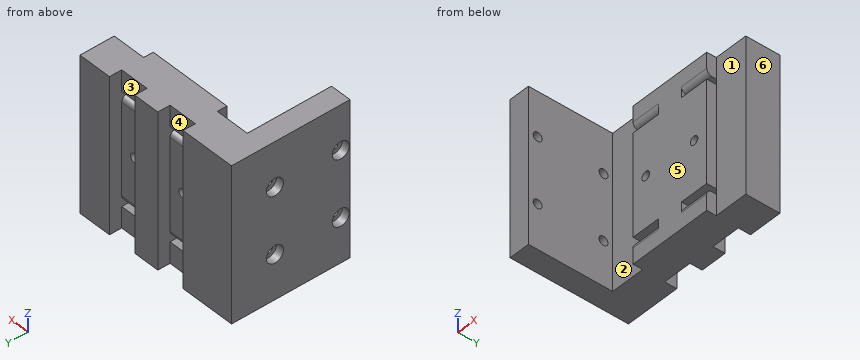
```python
from build123d import *

# Parameters (mm, degrees)
SKETCH1_W                       = 57.8
SKETCH1_H                       = 58.8
BOSS_EXTRUDE1_DEPTH             = 7
SKETCH5_W                       = 57.8
SKETCH5_H                       = 58.8
BOSS_EXTRUDE2_DEPTH             = 6
SKETCH6_W                       = 58.8
SKETCH6_H                       = 45
BOSS_EXTRUDE3_DEPTH             = 8
CBORE_FOR_M3_SHCS2_D            = 3.4
CBORE_FOR_M3_SHCS2_CBORE_D      = 6.5
CBORE_FOR_M3_SHCS2_CBORE_DEPTH  = 3
SKETCH10_W                      = 32
SKETCH10_H                      = 58.8
BOSS_EXTRUDE4_DEPTH             = 3.63
CUT_EXTRUDE1_START              = -4.63
SKETCH11_W                      = 32
SKETCH11_H                      = 8
CUT_EXTRUDE1_DEPTH              = 4.63
SKETCH12_W                      = 32
SKETCH12_H                      = 2
CUT_EXTRUDE2_DEPTH              = 63.094338711
SKETCH17_W                      = 32
SKETCH17_H                      = 58.8
CUT_EXTRUDE3_DEPTH              = 20
BOSS_EXTRUDE5_REACH             = 64.094
SKETCH18_W                      = 10
SKETCH18_H                      = 58.8
BOSS_EXTRUDE5_DIRECTION_2_REACH = 64.094
FILLET1_R                       = 2
M4X0_7_TAPPED_HOLE1_D           = 3.3


with BuildPart() as part:
    # Sketch1 → Boss-Extrude1 (new body)
    with BuildSketch(Plane(origin=(0, 0, 0), x_dir=(1, 0, 0), z_dir=(0, 1, 0))):
        Rectangle(SKETCH1_W, SKETCH1_H)
    extrude(amount=BOSS_EXTRUDE1_DEPTH)

    # Sketch5 → Boss-Extrude2 (add)
    with BuildSketch(Plane.XZ):
        Rectangle(SKETCH5_W, SKETCH5_H)
    extrude(amount=BOSS_EXTRUDE2_DEPTH)

    # Sketch6 → Boss-Extrude3 (add)
    with BuildSketch(Plane.ZY.offset(28.9)):
        with Locations((0, -15.5)):
            Rectangle(SKETCH6_W, SKETCH6_H)
    extrude(amount=BOSS_EXTRUDE3_DEPTH)

    # CBORE for M3 SHCS2 (through all)
    with Locations(Plane.ZY.offset(36.9)):
        with Locations((-12.5, -9.5), (12.5, -9.5), (12.5, -34.5), (-12.5, -34.5)):
            CounterBoreHole(CBORE_FOR_M3_SHCS2_D / 2, CBORE_FOR_M3_SHCS2_CBORE_D / 2, CBORE_FOR_M3_SHCS2_CBORE_DEPTH)

    # Sketch10 → Boss-Extrude4 (add)
    with BuildSketch(Plane.XZ.offset(6)):
        with Locations((0.1, 0)):
            Rectangle(SKETCH10_W, SKETCH10_H)
    extrude(amount=BOSS_EXTRUDE4_DEPTH)

    # Sketch11 → Cut-Extrude1 (cut)
    with BuildSketch(Plane(origin=(0, 7, 0), x_dir=(1, 0, 0), z_dir=(0, 1, 0)).offset(CUT_EXTRUDE1_START)):
        with Locations((0.1, -25.4)):
            Rectangle(SKETCH11_W, SKETCH11_H)
    cut_extrude1 = extrude(amount=CUT_EXTRUDE1_DEPTH, mode=Mode.SUBTRACT)

    # Sketch12 → Cut-Extrude2 (cut, symmetric)
    with BuildSketch(Plane(origin=(0, 2.37, 0), x_dir=(1, 0, 0), z_dir=(0, 1, 0))):
        with Locations((0.1, -20.4)):
            Rectangle(SKETCH12_W, SKETCH12_H)
    cut_extrude2 = extrude(amount=CUT_EXTRUDE2_DEPTH, both=True, mode=Mode.SUBTRACT)

    # Mirror1: Cut-Extrude1, Cut-Extrude2 across plane
    add(cut_extrude1.mirror(Plane.XY), mode=Mode.SUBTRACT)
    add(cut_extrude2.mirror(Plane.XY), mode=Mode.SUBTRACT)

    # Sketch17 → Cut-Extrude3 (cut)
    with BuildSketch(Plane(origin=(0, 2.37, 0), x_dir=(1, 0, 0), z_dir=(0, 1, 0))):
        with Locations((0.1, 0)):
            Rectangle(SKETCH17_W, SKETCH17_H)
    extrude(amount=CUT_EXTRUDE3_DEPTH, mode=Mode.SUBTRACT)

    # Boss-Extrude5: up to this face of the body (flat: up to its plane)
    boss_extrude5_end = Plane(part.part.faces().sort_by_distance((22.5, 7, 0))[0])
    # Sketch18 → Boss-Extrude5 (add, up to the picked face)
    with BuildSketch(Plane(origin=(0, 2.37, 0), x_dir=(1, 0, 0), z_dir=(0, 1, 0)), mode=Mode.PRIVATE) as boss_extrude5_sk1:
        with Locations((0.1, 0)):
            Rectangle(SKETCH18_W, SKETCH18_H)
    boss_extrude5_tool1 = split(extrude(boss_extrude5_sk1.sketch, amount=BOSS_EXTRUDE5_REACH, mode=Mode.PRIVATE), bisect_by=boss_extrude5_end, keep=Keep.BOTH, mode=Mode.PRIVATE)
    add(boss_extrude5_tool1.solids().sort_by(Axis((0.1, 2.37, 0), (0, 1, 0)))[0])

    # Boss-Extrude5 direction 2: up to this face of the body (flat: up to its plane)
    boss_extrude5_direction_2_end = Plane(part.part.faces().sort_by_distance((0.1, -9.63, 0))[0])
    # Sketch18 → Boss-Extrude5 direction 2 (add, up to the picked face)
    with BuildSketch(Plane(origin=(0, 2.37, 0), x_dir=(1, 0, 0), z_dir=(0, 1, 0)), mode=Mode.PRIVATE) as boss_extrude5_direction_2_sk1:
        with Locations((0.1, 0)):
            Rectangle(SKETCH18_W, SKETCH18_H)
    boss_extrude5_direction_2_tool1 = split(extrude(boss_extrude5_direction_2_sk1.sketch, amount=-BOSS_EXTRUDE5_DIRECTION_2_REACH, mode=Mode.PRIVATE), bisect_by=boss_extrude5_direction_2_end, keep=Keep.BOTH, mode=Mode.PRIVATE)
    add(boss_extrude5_direction_2_tool1.solids().sort_by(Axis((0.1, 2.37, 0), (0, -1, 0)))[0])

    # Fillet1
    fillet1_edges = [part.edges().sort_by_distance(p)[0] for p in [
        (10.6, -9.63, 21.4),
        (10.6, -9.63, -21.4),
        (10.6, 2.37, -19.4),
        (10.6, 2.37, 19.4),
        (-10.4, 2.37, -19.4),
        (-10.4, 2.37, 19.4),
        (-10.4, -9.63, -21.4),
        (-10.4, -9.63, 21.4),
    ]]
    fillet(fillet1_edges, radius=FILLET1_R)

    # M4x0.7 Tapped Hole1 (through all)
    with Locations(Plane(origin=(0, 2.37, 0), x_dir=(1, 0, 0), z_dir=(0, 1, 0))):
        with Locations((-10.4, 0), (10.6, 0)):
            Hole(M4X0_7_TAPPED_HOLE1_D / 2)


solid = part.part
```
For this review, take the finished solid that the model builds, in its own axes (mm). Face numbers are marked on the shaded views. A direction names the side the tool comes from. Coordinates: 2 decimals unless noted, no trailing zeros. Loops run counter-clockwise (first coordinate to the right, second up) from the corner with the lowest first, then second, coordinate; pieces in that order, holes last. Notation, with made-up numbers: (70.5, -32.5) - (117.5, -32.5) arc R15 ccw to (117.5, -28.5) - close; hole circle Ø8 at (16, -30). An arc over 180 degrees is marked (long way). Use one line per item in the form item = value. Start each with the question number.
1) Take a section at C-C (y = -17.5). State the section outline as (x, z) points.
2) For pin 1 (5 mm diameter, centred on y = -11, z = -13.5, fed in from -X); pin 2 (4 mm diameter, centred on x = 21, z = 20, fed in from -Y); pin 3 (10 mm diameter, centred on x = 8, z = 22, fed in from -Y); pin 4 (10 mm diameter, centred on y = -28.5, z = 19, fed in from +X), all flat-tipped, find the tip position at first contact; note any pin that passes through.
3) Take a section at D-D (z = 24.5). State the section outline as (x, y) points, plus the area to 3 significant figures.
4) Take a section at A-A (z = -12.5). State how many separate pieces and enclosed holes the cut face has, plus the area to 3 significant figures.
5) For the marked faces 1, 2 and 3, list the 3-axis set-ups (+Z, -Z, +X, -X, +Y, -Y) from which the entire face can be reached by the end or side of a thin tool; tool diameter is ignored.
6) To check wall thickness, follow probe 1 along Z at (x, y) = (-7, -5.5); probe 2 along Y at (x, z) = (-35.1, -12.5); probe 3 along Y at (x, z) = (-30.8, -12.5). State the ranges of each line that lie inside material, in increasing order. Write a range as from..to.
7) Take a section at B-B (x = -10.4). State the section outline as (y, z) points.
8) Draft analysis for pull direction X (two halves, no side actions). For the marked faces 4, 5 and 6, state which applies: released by +X, released by -X, zero draft, split by the parting line, or undercut.
From the geometry:
q1.outline = (-36.9, -29.4) - (-28.9, -29.4) - (-28.9, 29.4) - (-36.9, 29.4) - close
q2.pin_1 = -36.9
q2.pin_2 = -6
q2.pin_3 = -9.63
q2.pin_4 = -28.9
q3.outline = (-36.9, -38) - (-28.9, -38) - (-28.9, -6) - (-15.9, -6) - (-15.9, -9.63) - (16.1, -9.63) - (16.1, -6) - (28.9, -6) - (28.9, 7) - (16.1, 7) - (16.1, 2.37) - (5.1, 2.37) - (5.1, 7) - (-4.9, 7) - (-4.9, 2.37) - (-15.9, 2.37) - (-15.9, 7) - (-36.9, 7) - close
q3.area = 1,130 mm2
q4.separate_pieces = 3
q4.enclosed_holes = 0
q4.area = 1,050 mm2
q5.face_1 = +Z, -Z, +X, -Y
q5.face_2 = +Z, -Z, -Y
q5.face_3 = +Z, -Z, +Y
q6.probe_1 = -29.4..-21.4, -19.4..19.4, 21.4..29.4
q6.probe_2 = -38..-37.75, -31.25..-12.75, -6.25..7
q6.probe_3 = -38..-36.2, -32.8..-11.2, -7.8..7
q7.outline = (-9.63, -29.4) - (2.37, -29.4) - (2.37, -21.4) - (-7.63, -21.4) arc R2 ccw to (-9.63, -23.4) - close; (-9.63, -19.4) - (0.37, -19.4) arc R2 ccw to (2.37, -17.4) - (2.37, -1.65) - (-9.63, -1.65) - close; (-9.63, 1.65) - (2.37, 1.65) - (2.37, 17.4) arc R2 ccw to (0.37, 19.4) - (-9.63, 19.4) - close; (-9.63, 23.4) arc R2 ccw to (-7.63, 21.4) - (2.37, 21.4) - (2.37, 29.4) - (-9.63, 29.4) - close
q8.face_4 = undercut
q8.face_5 = zero draft
q8.face_6 = released by +X
